Can you work these out from the model? Positions are in its coordinate system, mm. A direction names the side the tool comes from. Round coordinates to 2 decimals unless told otherwise and drop trailing zeros. Order: outer loops, then holes, each group sorted by start corner. A loop starts at its lowest first (then second) coordinate and runs counter-clockwise, first axis right, second up.
from build123d import *

# Parameters (mm, degrees)
SKETCH1_W                    = 41.148
SKETCH1_H                    = 44.45
BOSS_EXTRUDE1_DEPTH          = 6.35
FILLET1_R                    = 2.54
SKETCH2_R                    = 11.43
CUT_EXTRUDE1_DEPTH           = 7.35
F_25_0_1495_DIAMETER_HOLE1_D = 3.7973
F_10_32_TAPPED_HOLE2_D       = 4.0386
CUT_EXTRUDE2_DEPTH           = 3.81


with BuildPart() as part:
    # Sketch1 → Boss-Extrude1 (new body)
    with BuildSketch(Plane(origin=(0, 0, 0), x_dir=(1, 0, 0), z_dir=(0, 1, 0))):
        Rectangle(SKETCH1_W, SKETCH1_H)
    extrude(amount=BOSS_EXTRUDE1_DEPTH)

    # Fillet1
    fillet1_edges = [part.edges().sort_by_distance(p)[0] for p in [
        (-20.574, 3.175, -22.225),
        (20.574, 3.175, -22.225),
        (20.574, 3.175, 22.225),
        (-20.574, 3.175, 22.225),
    ]]
    fillet(fillet1_edges, radius=FILLET1_R)

    # Sketch2 → Cut-Extrude1 (cut, through all)
    with BuildSketch(Plane(origin=(0, 6.35, 0), x_dir=(1, 0, 0), z_dir=(0, 1, 0))):
        Circle(SKETCH2_R)
    extrude(amount=-CUT_EXTRUDE1_DEPTH, mode=Mode.SUBTRACT)

    # #25 (0.1495) Diameter Hole1 (through all)
    with Locations(Plane(origin=(-17.399, 6.35, -16.645384286), x_dir=(0, 0, 1), z_dir=(0, 1, 0))):
        with Locations((0, 0), (0, 34.798), (26.940768363, 34.798), (26.940768363, 0)):
            Hole(F_25_0_1495_DIAMETER_HOLE1_D / 2)

    # #10-32 Tapped Hole2 (through all)
    with Locations(Plane(origin=(-15.133967136, 6.35, -8.7376), x_dir=(0, 0, 1), z_dir=(0, 1, 0))):
        with Locations((0, 0), (0, 30.267934272), (26.2128, 15.133967136)):
            Hole(F_10_32_TAPPED_HOLE2_D / 2)

    # Sketch9 → Cut-Extrude2 (cut)
    with BuildSketch(Plane(origin=(0, 6.35, 0), x_dir=(1, 0, 0), z_dir=(0, 1, 0))):
        with BuildLine():
            Line((-20.574, 13.470384286), (-20.574, 19.820384286))
            Line((-20.574, 19.820384286), (-17.399, 19.820384286))
            ThreePointArc((-17.399, 19.820384286), (-14.224, 16.645384286), (-17.399, 13.470384286))
            Line((-17.399, 13.470384286), (-20.574, 13.470384286))
        make_face()
        with BuildLine():
            Line((17.399, 13.470384286), (20.574, 13.470384286))
            Line((20.574, 13.470384286), (20.574, 19.820384286))
            Line((20.574, 19.820384286), (17.399, 19.820384286))
            ThreePointArc((17.399, 19.820384286), (14.224, 16.645384286), (17.399, 13.470384286))
        make_face()
        with BuildLine():
            Line((20.574, -7.120384286), (20.574, -13.470384286))
            Line((20.574, -13.470384286), (17.399, -13.470384286))
            ThreePointArc((17.399, -13.470384286), (14.224, -10.295384286), (17.399, -7.120384286))
            Line((17.399, -7.120384286), (20.574, -7.120384286))
        make_face()
        with BuildLine():
            Line((-17.399, -7.120384286), (-20.574, -7.120384286))
            Line((-20.574, -7.120384286), (-20.574, -13.470384286))
            Line((-20.574, -13.470384286), (-17.399, -13.470384286))
            ThreePointArc((-17.399, -13.470384286), (-14.224, -10.295384286), (-17.399, -7.120384286))
        make_face()
    extrude(amount=-CUT_EXTRUDE2_DEPTH, mode=Mode.SUBTRACT)


solid = part.part
(1) I want a section at D-D, the plane z = -9. List the corners of the cut face in (x, y) for me, plus the area to 3 significant figures.
(2) On a 3-axis mill with a long thin cutter (end or side, diameter ignored), from which of +Z, -Z, +X, -X, +Y, -Y can I reach the whole of each face in a straight line? I mean faces 1 (the face through (-19.85, 3.22, 21.46)), 2 (the face through (-14.225, 4.472, 10.365)), 3 (the face through (19, 4, -19.82)). Say none if no direction works.
(3) If we mould it in two halves opening along Z, with no side actions, what happens to faces 4 (the face through (9, 6.35, -10)), 5 (the face through (-19, 2.54, -15)), 6 (the face through (0, 3, 22.225))? For each: pulls with the +Z half, pulls with the -Z half, needs draft (parallel to the pull), parting line crosses it, or undercut.
(4) I want a section at B-B, the plane z = 0. List the corners of the cut face in (x, y) for me.
(5) I want a section at C-C, the plane y = 4.75. List the corners of the cut face in (x, z) for me (3 decimals), plus the area to 3 significant figures.
(6) I want a section at A-A, the plane x = 0. Give the number of separate pieces and of enclosed holes in the cut face, plus the area to 3 significant figures.
(7) I'm going to push flat-ended pins straight in: pin 1 Ø2.5 at (x, y) = (-18.5, 4.5) entering from +Z (3 decimals); pin 2 Ø1.9 at (x, z) = (-16.5, 11.5) entering from +Y; pin 3 Ø1.6 at (x, y) = (19.5, 3.5) entering from -Z. Where does each tip first touch, or does it pass through?
(8) Please list where these lines run through material, in increasing order: probe 1 along Z at (x, y) = (18.5, 1); probe 2 along Z at (x, y) = (-16.5, 3) (3 decimals); probe 3 along Z at (x, y) = (-1.5, 3.25) (3 decimals).
Ans:
1. outline: (-20.57, 0) - (-17.14, 0) - (-17.14, 6.35) - (-20.57, 6.35) - close; (-13.13, 0) - (-7.05, 0) - (-7.05, 6.35) - (-13.13, 6.35) - close; (7.05, 0) - (13.13, 0) - (13.13, 6.35) - (7.05, 6.35) - close; (17.14, 0) - (20.57, 0) - (20.57, 6.35) - (17.14, 6.35) - close
1. area: 121 mm2
2. face 1: +Z, -X, +Y, -Y
2. face 2: -X, +Y
2. face 3: +X, +Y
3. face 4: needs draft
3. face 5: undercut
3. face 6: pulls with the +Z half
4. outline: (-20.57, 0) - (-11.43, 0) - (-11.43, 6.35) - (-20.57, 6.35) - close; (11.43, 0) - (20.57, 0) - (20.57, 6.35) - (11.43, 6.35) - close
5. outline: (-20.574, -13.47) - (-17.399, -13.47) arc R3.175 cw to (-17.399, -19.82) - (-20.57, -19.82) arc R2.54 ccw to (-18.034, -22.225) - (18.034, -22.225) arc R2.54 ccw to (20.57, -19.82) - (17.399, -19.82) arc R3.175 cw to (17.399, -13.47) - (20.574, -13.47) - (20.574, 7.12) - (17.399, 7.12) arc R3.175 cw to (17.399, 13.47) - (20.574, 13.47) - (20.574, 19.685) arc R2.54 ccw to (18.034, 22.225) - (-18.034, 22.225) arc R2.54 ccw to (-20.574, 19.685) - (-20.574, 13.47) - (-17.399, 13.47) arc R3.175 cw to (-17.399, 7.12) - (-20.574, 7.12) - close; hole circle Ø4.039 at (-15.134, -8.738); hole circle Ø22.86 at (0, 0); hole circle Ø4.039 at (0, 17.475); hole circle Ø4.039 at (15.134, -8.738)
5. area: 1,230 mm2
6. separate pieces: 3
6. enclosed holes: 0
6. area: 111 mm2
7. pin 1: stops at z = 22.225
7. pin 2: stops at y = 2.54
7. pin 3: stops at z = -22.14
8. probe 1: z = -22.18 to -18.19, -15.1 to 8.75, 11.84 to 22.18
8. probe 2: z = -22.225 to -19.69, -13.6 to -10.225, -7.25 to 7.25, 13.34 to 22.225
8. probe 3: z = -22.225 to -11.331, 11.331 to 16.123, 18.827 to 22.225
